```python
from build123d import *

# Parameters (mm, degrees)
SKETCH1_W           = 30
SKETCH1_H           = 15
BOSS_EXTRUDE1_DEPTH = 1.2
SKETCH2_W           = 1.2
SKETCH2_H           = 15
CUT_EXTRUDE1_DEPTH  = 0.02
SKETCH3_W           = 12
SKETCH3_H           = 12.6
BOSS_EXTRUDE2_DEPTH = 0.8
SKETCH4_W           = 12
SKETCH4_H           = 12.6
BOSS_EXTRUDE3_DEPTH = 0.8


with BuildPart() as part:
    # Sketch1 → Boss-Extrude1 (new body)
    with BuildSketch(Plane(origin=(0, 0, 0), x_dir=(1, 0, 0), z_dir=(0, 1, 0))):
        Rectangle(SKETCH1_W, SKETCH1_H)
    extrude(amount=BOSS_EXTRUDE1_DEPTH)

    # Sketch2 → Cut-Extrude1 (cut)
    with BuildSketch(Plane(origin=(0, 1.2, 0), x_dir=(1, 0, 0), z_dir=(0, 1, 0))):
        Rectangle(SKETCH2_W, SKETCH2_H)
    extrude(amount=-CUT_EXTRUDE1_DEPTH, mode=Mode.SUBTRACT)

    # Sketch3 → Boss-Extrude2 (add)
    with BuildSketch(Plane(origin=(0, 1.2, 0), x_dir=(1, 0, 0), z_dir=(0, 1, 0))):
        with Locations((-7.8, 0)):
            Rectangle(SKETCH3_W, SKETCH3_H)
    extrude(amount=BOSS_EXTRUDE2_DEPTH)

    # Sketch4 → Boss-Extrude3 (add)
    with BuildSketch(Plane(origin=(0, 1.2, 0), x_dir=(1, 0, 0), z_dir=(0, 1, 0))):
        with Locations((7.8, 0)):
            Rectangle(SKETCH4_W, SKETCH4_H)
    extrude(amount=BOSS_EXTRUDE3_DEPTH)


solid = part.part
```
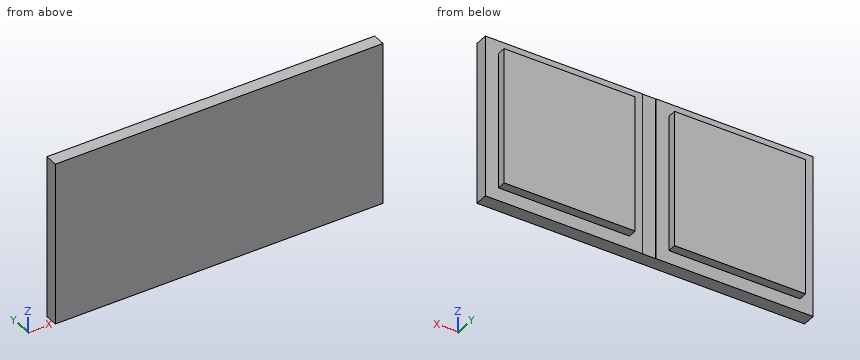
Read the model definition and answer for the solid it produces. Units are mm, in the model's axes. Round coordinates to 2 decimals unless told otherwise and drop trailing zeros. Loops run counter-clockwise (first coordinate to the right, second up) from the corner with the lowest first, then second, coordinate; pieces in that order, holes last. Notation, with made-up numbers: (7.5, 80) -> (28.5, 80) arc R15 ccw to (28.5, 90) -> close; hole circle Ø9 at (69.5, 9.25). An arc over 180 degrees is marked (long way). One line per item, written item: value.
1) Flat-ended cylindrical pins translate along their axes: P1, Ø1, axis at x = 0, z = 0.5, coming from the +Y side; P2, Ø0.6, axis at x = 6.5, y = 2, coming from the +Z side; P3, Ø0.6, axis at x = 8.5, y = 2, coming from the -Z side. Find the tip coordinate at first contact, or state that the pin passes through.
Answer list:
P1: stops at y = 1.18
P2: stops at z = 6.3
P3: stops at z = -6.3
2) A cutting plane is placed at C-C (x = 11.75). Determine the outline of the cut face in (y, z), and give its area (3 significant figures).
Answer list:
outline: (0, -7.5) -> (1.2, -7.5) -> (1.2, -6.3) -> (2, -6.3) -> (2, 6.3) -> (1.2, 6.3) -> (1.2, 7.5) -> (0, 7.5) -> close
area: 28.1 mm²
3) Consider L1, parallel to X at y = 1.65, z = 3; L2, parallel to Z at x = 11.25, y = 1.3; L3, parallel to Y at x = -1.5, z = 0.75. Determine where each line is inside the solid, lowest interval first. Write a range as [from, to].
Answer list:
L1: x = [-13.8, -1.8], [1.8, 13.8]
L2: z = [-6.3, 6.3]
L3: y = [0, 1.2]
4) A cutting plane is placed at A-A (y = 1.5). Determine the outline of the cut face in (x, z), and give its area (3 significant figures).
Answer list:
outline: (-13.8, -6.3) -> (-1.8, -6.3) -> (-1.8, 6.3) -> (-13.8, 6.3) -> close; (1.8, -6.3) -> (13.8, -6.3) -> (13.8, 6.3) -> (1.8, 6.3) -> close
area: 302 mm²
